Geometry: see drawing. Coordinates: mm, zero at the bounding-box minimum. A direction names the side the tool comes from. Give positions to 0.01 mm unless a question says otherwise; leave off trailing zeros. Order: outer loops, then holes, each group sorted by start corner. A loop starts at its lowest first (then second) coordinate and runs counter-clockwise, first axis right, second up. Notation, with made-up numbers: (64, -21) - (99, -21) arc R7 ccw to (99, -14) - close; hole circle Ø5 at (84.5, 35). An arc over 180 degrees is marked (long way). One line per item, written item: value.
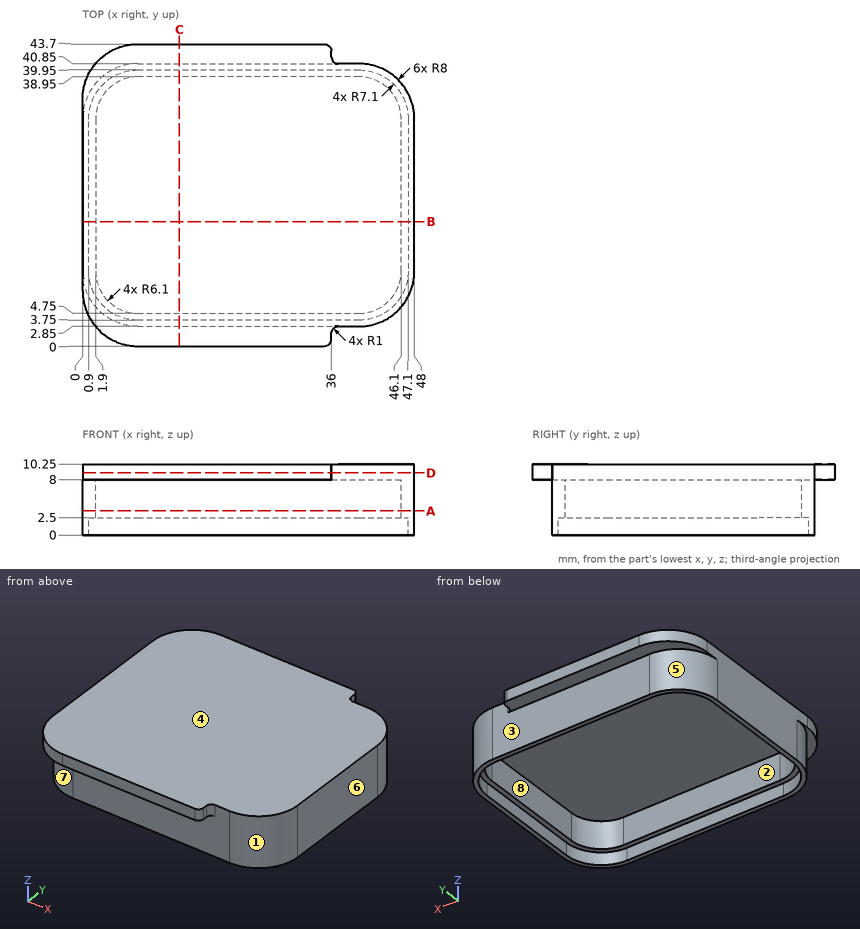
1) Mould query, pull axis X, two halves, no side actions, for the marked faces 1, 2 and 3. Classes: released by +X, released by -X, zero draft, split by the parting line, or undercut.
Answers below:
face 1: released by +X
face 2: undercut
face 3: zero draft
2) Section B-B, the plane y = 18. Return loops of the section in (x, z), then the cut area to 3 significant figures.
Answers below:
outline: (0, 0) - (0.9, 0) - (0.9, 2.5) - (1.9, 2.5) - (1.9, 8) - (46.1, 8) - (46.1, 2.5) - (47.1, 2.5) - (47.1, 0) - (48, 0) - (48, 10.25) - (0, 10.25) - close
area: 133 mm^2
3) First-contact query: pin 1 (1.5 mm diameter, centred on x = 40, y = 16.5, fed in from -Z); pin 2 (6 mm diameter, centred on x = 16, z = 4, fed in from -Y); pin 3 (3 mm diameter, centred on x = 19, y = 37.5, fed in from -Z). Flat tips, straight axial feed; report the tip coordinate or a pass-through.
Answers below:
pin 1: z = 8
pin 2: y = 2.85
pin 3: z = 2.5
4) Material intervals for line 1 along Y through (x, z) = (27, 3.5); line 2 along X through (y, z) = (23, 2.75); line 3 along Z through (x, y) = (8, 42), sorted ascending.
Answers below:
line 1: 2.85 to 4.75, 38.95 to 40.85
line 2: 0 to 1.9, 46.1 to 48
line 3: 8 to 10.25
5) Section C-C, the plane x = 14. Return loops of the section in (y, z).
Answers below:
outline: (0, 8) - (2.85, 8) - (2.85, 0) - (3.75, 0) - (3.75, 2.5) - (4.75, 2.5) - (4.75, 8) - (38.95, 8) - (38.95, 2.5) - (39.95, 2.5) - (39.95, 0) - (40.85, 0) - (40.85, 8) - (43.7, 8) - (43.7, 10.25) - (0, 10.25) - close
6) Section A-A, the plane z = 3.5. Return loops of the section in (x, y), then the cut area to 3 significant figures.
Answers below:
outline: (0, 10.85) arc R8 ccw to (8, 2.85) - (40, 2.85) arc R8 ccw to (48, 10.85) - (48, 32.85) arc R8 ccw to (40, 40.85) - (8, 40.85) arc R8 ccw to (0, 32.85) - close; hole (1.9, 10.85) arc R6.1 ccw to (8, 4.75) - (40, 4.75) arc R6.1 ccw to (46.1, 10.85) - (46.1, 32.85) arc R6.1 ccw to (40, 38.95) - (8, 38.95) arc R6.1 ccw to (1.9, 32.85) - close
area: 289 mm^2
7) Set-up query: the marked faces 4, 5, 6, 7 and 8. Return all of +Z, -Z, +X, -X, +Y, -Y with unobstructed straight access to the full face (end or side cutting, diameter ignored); none if empty.
Answers below:
face 4: +Z, +X, -X, +Y, -Y
face 5: -Z, -X, +Y
face 6: +Z, -Z, +X, +Y, -Y
face 7: -Z, -X, -Y
face 8: -Z
8) Section D-D, the plane z = 9. Return loops of the section in (x, y).
Answers below:
outline: (0, 8) arc R8 ccw to (8, 0) - (35, 0) arc R1 ccw to (36, 1) - (36, 1.85) arc R1 cw to (37, 2.85) - (40, 2.85) arc R8 ccw to (48, 10.85) - (48, 32.85) arc R8 ccw to (40, 40.85) - (37, 40.85) arc R1 cw to (36, 41.85) - (36, 42.7) arc R1 ccw to (35, 43.7) - (8, 43.7) arc R8 ccw to (0, 35.7) - close
